Geometry: final body of the model. Coordinates: model frame, mm. Face numbers are marked on the shaded views. A direction names the side the tool comes from. Coordinates: 2 decimals unless noted, no trailing zeros. Loops run counter-clockwise (first coordinate to the right, second up) from the corner with the lowest first, then second, coordinate; pieces in that order, holes last. Notation, with made-up numbers: (39.5, 63) - (45.5, 63) arc R21 cw to (45.5, 77) - close; hole circle Ø9 at (-30.5, -35.5). An arc over 180 degrees is marked (long way). Put each result on its own line as item: value. Start each with the question number.
1) Draft query along X for the marked faces 1, 2, 3 and 4. Return one class per face: +X half, -X half, draft (parallel to the pull), parting line (faces both ways), or undercut.
2) Section C-C on x = -6.25. Output: boundary loops of the cut face in (y, z), and give its area (3 significant figures).
3) Reachability of the marked faces 5 and 6 from +Z, -Z, +X, -X, +Y, -Y: full face, straight path, thin tool, end or side. Return the list, or none.
4) Contact query for flat-ended pins moving along their axis: pin 1 Ø6 at (x, y) = (-1.5, 5) entering from -Z; pin 2 Ø3 at (x, z) = (-8.5, 5) entering from -Y; pin 3 Ø3 at (x, z) = (-7.5, 9) entering from -Y. Output: stop coordinate, or through.
5) Material intervals for line 1 along Y through (x, z) = (-4, 0); line 2 along Y through (x, z) = (-2.25, 0); line 3 along X through (y, z) = (11.5, -12.5), sorted ascending. Write a range as from..to.
6) Section A-A on z = 0. Output: boundary loops of the cut face in (x, y).
7) Section D-D on x = -9.5. Output: boundary loops of the cut face in (y, z), and give its area (3 significant figures).
```python
from build123d import *

# Parameters (mm, degrees)
SKETCH3_R          = 5.08
CUT_EXTRUDE1_DEPTH = 29.638898375


with BuildPart() as part:
    # Sketch2 → Revolve1 (revolve)
    with BuildSketch(Plane.XY, mode=Mode.PRIVATE) as revolve1_sk:
        Polygon((0, 0), (-10.16, 0), (-10.16, 17.209662464), (-8.436082504, 18.933579959), (-7.4549, 18.933579959), (-7.4549, 15.898279959), (-2.7051, 15.898279959), (-2.7051, 18.933579959), (-1.723917496, 18.933579959), (0, 17.209662464), align=None)
    revolve(revolve1_sk.sketch.rotate(Axis((0, 0, 0), (-1, 0, 0)), 90), axis=Axis((0, 0, 0), (-1, 0, 0)))

    # Sketch3 → Cut-Extrude1 (cut, through all)
    with BuildSketch(Plane(origin=(0, 0, 0), x_dir=(0, 0, -1), z_dir=(1, 0, 0))):
        Circle(SKETCH3_R)
    extrude(amount=-CUT_EXTRUDE1_DEPTH, mode=Mode.SUBTRACT)


solid = part.part
```
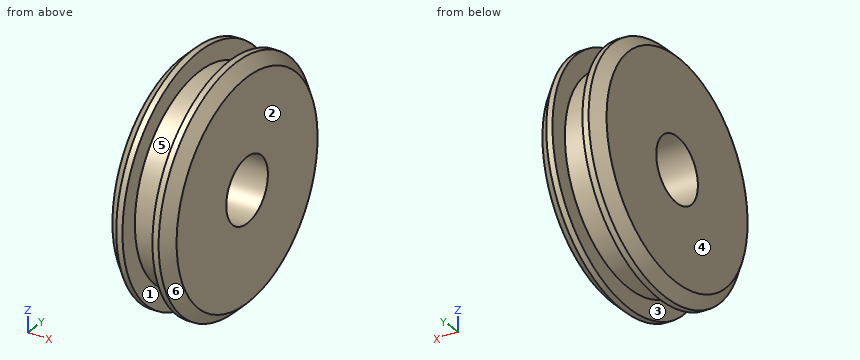
Answer block:
1. face 1: undercut
1. face 2: +X half
1. face 3: undercut
1. face 4: -X half
2. outline: circle Ø31.8 at (0, 0); hole circle Ø10.16 at (0, 0)
2. area: 713 mm²
3. face 5: none
3. face 6: +X
4. pin 1: stops at z = -18.83
4. pin 2: stops at y = -18.61
4. pin 3: stops at y = -17.38
5. line 1: y = -15.9..-5.08, 5.08..15.9
5. line 2: y = -18.93..-5.08, 5.08..18.93
5. line 3: x = -10.16..-7.45, -2.71..0
6. outline: (-10.16, -17.21) - (-8.44, -18.93) - (-7.45, -18.93) - (-7.45, -15.9) - (-2.71, -15.9) - (-2.71, -18.93) - (-1.72, -18.93) - (0, -17.21) - (0, -5.08) - (-10.16, -5.08) - close; (-10.16, 5.08) - (0, 5.08) - (0, 17.21) - (-1.72, 18.93) - (-2.71, 18.93) - (-2.71, 15.9) - (-7.45, 15.9) - (-7.45, 18.93) - (-8.44, 18.93) - (-10.16, 17.21) - close
7. outline: circle Ø35.74 at (0, 0); hole circle Ø10.16 at (0, 0)
7. area: 922 mm²
